Could you check a few things on this model? Use its own coordinates, in mm. A direction names the side the tool comes from. Coordinates: 2 decimals unless noted, no trailing zeros. Loops run counter-clockwise (first coordinate to the right, second up) from the corner with the lowest first, then second, coordinate; pieces in that order, holes last. Notation, with made-up numbers: (-14, 60.5) -> (44, 60.5) arc R22 ccw to (44, 89.5) -> close; hole circle Ø9 at (-26.75, -5). An arc over 180 degrees is marked (long way). One line per question, with ' | ' between items.
Autodesk Fusion 360 part; units mm, degrees
sketch "Sketch2" plane through (0, 0, 0) normal (0, 0, 1) x (1, 0, 0)
  line L0 (0, 0) -> (146.5, 0)
  line L1 (146.5, 0) -> (146.5, 57.5)
  line L2 (146.5, 57.5) -> (0, 57.5)
  line L3 (0, 57.5) -> (0, 0)
  line L4 (69.25, 0) -> (77.25, 0)
  line L5 (77.25, 0) -> (77.25, -8)
  line L6 (77.25, -8) -> (69.25, -8)
  line L7 (69.25, -8) -> (69.25, 0)
  line L8 (146.5, 24.75) -> (146.5, 32.75)
  line L9 (146.5, 32.75) -> (154.5, 32.75)
  line L10 (154.5, 32.75) -> (154.5, 24.75)
  line L11 (154.5, 24.75) -> (146.5, 24.75)
  line L12 (73.25, 57.5) -> (73.25, 0) construction
  line L13 (146.5, 28.75) -> (154.5, 28.75) construction
  line L14 (150.5, 32.75) -> (150.5, 24.75) construction
  circle A0 centre (150.5, 28.75) radius 1.75
  line L15 (-8, 24.75) -> (0, 24.75)
  line L16 (-8, 32.75) -> (-8, 24.75)
  line L17 (0, 32.75) -> (-8, 32.75)
  circle A1 centre (-4, 28.75) radius 1.75
  line L18 (69.25, -4) -> (77.25, -4) construction
  line L19 (73.25, 0) -> (73.25, -8) construction
  circle A2 centre (73.25, -4) radius 1.75
  point P0 (73.25, 0)
  point P1 (146.5, 28.75)
  point P2 (-8, 28.75)
  dimension "d8" = 146.5
  dimension "d9" = 57.5
  dimension "d12" = 8
  dimension "d13" = 8
  dimension "d14" = 8
  dimension "d15" = 8
  dimension "d16" = 8
  dimension "d17" = 3.5
  dimension "d18" = 3.5
extrude "Extrude1" add sketch "Sketch2" along normal blind 3
fillet "Fillet1" radius 1.5 12 edges at (77.25, 0, 1.5) (77.25, -8, 1.5) (69.25, -8, 1.5) (69.25, 0, 1.5) (0, 24.75, 1.5) (-8, 24.75, 1.5) (-8, 32.75, 1.5) (0, 32.75, 1.5) (154.5, 32.75, 1.5) (146.5, 32.75, 1.5) (146.5, 24.75, 1.5) (154.5, 24.75, 1.5)
sketch "Sketch3" plane through (0, 0, 3) normal (0, 0, 1) x (-1, 0, 0)
  arc A0 (-153, -24.75) -> (-154.5, -26.25) centre (-153, -26.25) ccw
  line L0 (-154.5, -26.25) -> (-154.5, -31.25)
  arc A1 (-154.5, -31.25) -> (-153, -32.75) centre (-153, -31.25) ccw
  line L1 (-153, -32.75) -> (-148, -32.75)
  arc A2 (-146.5, -34.25) -> (-148, -32.75) centre (-148, -34.25) ccw
  line L2 (-146.5, -34.25) -> (-146.5, -57.5)
  line L3 (-146.5, -57.5) -> (0, -57.5)
  line L4 (0, -57.5) -> (0, -34.25)
  arc A3 (1.5, -32.75) -> (0, -34.25) centre (1.5, -34.25) ccw
  line L5 (1.5, -32.75) -> (6.5, -32.75)
  arc A4 (6.5, -32.75) -> (8, -31.25) centre (6.5, -31.25) ccw
  line L6 (8, -31.25) -> (8, -26.25)
  arc A5 (8, -26.25) -> (6.5, -24.75) centre (6.5, -26.25) ccw
  line L7 (6.5, -24.75) -> (1.5, -24.75)
  arc A6 (0, -23.25) -> (1.5, -24.75) centre (1.5, -23.25) ccw
  line L8 (0, -23.25) -> (0, 0)
  line L9 (0, 0) -> (-67.75, 0)
  arc A7 (-69.25, 1.5) -> (-67.75, 0) centre (-67.75, 1.5) ccw
  line L10 (-69.25, 1.5) -> (-69.25, 6.5)
  arc A8 (-69.25, 6.5) -> (-70.75, 8) centre (-70.75, 6.5) ccw
  line L11 (-70.75, 8) -> (-75.75, 8)
  arc A9 (-75.75, 8) -> (-77.25, 6.5) centre (-75.75, 6.5) ccw
  line L12 (-77.25, 6.5) -> (-77.25, 1.5)
  arc A10 (-78.75, 0) -> (-77.25, 1.5) centre (-78.75, 1.5) ccw
  line L13 (-78.75, 0) -> (-146.5, 0)
  line L14 (-146.5, 0) -> (-146.5, -23.25)
  arc A11 (-148, -24.75) -> (-146.5, -23.25) centre (-148, -23.25) ccw
  line L15 (-148, -24.75) -> (-153, -24.75)
  circle A12 centre (-150.5, -28.75) radius 1.75
  circle A13 centre (4, -28.75) radius 1.75
  circle A14 centre (-73.25, 4) radius 1.75
  line L16 (0, -2.5) -> (-146.5, -2.5) construction
  line L17 (-54.25, -2.5) -> (-92.25, -2.5)
  line L18 (-92.25, -2.5) -> (-92.25, 0)
  line L19 (-54.25, -2.5) -> (-54.25, 0)
  line L20 (-54.25, 0) -> (-92.25, 0)
  line L21 (-144, -57) -> (-144, 0) construction
  line L22 (-144, -13.5) -> (-144, -43.5)
  line L23 (-144, -43.5) -> (-146.5, -43.5)
  line L24 (-144, -13.5) -> (-146.5, -13.5)
  line L25 (-146.5, -13.5) -> (-146.5, -43.5)
  line L26 (-73.25, -57.5) -> (-73.25, 0) construction
  line L27 (-2.5, -13.5) -> (0, -13.5)
  line L28 (0, -13.5) -> (0, -43.5)
  line L29 (-2.5, -43.5) -> (0, -43.5)
  line L30 (-2.5, -13.5) -> (-2.5, -43.5)
  line L31 (0, -55) -> (-146.5, -55) construction
  line L32 (-50.75, -55) -> (-95.75, -55)
  line L33 (-95.75, -55) -> (-95.75, -57.5)
  line L34 (-50.75, -55) -> (-50.75, -57.5)
  line L35 (-50.75, -57.5) -> (-95.75, -57.5)
  line L36 (-70.75, -55) -> (-75.75, -55)
  line L37 (-75.75, -55) -> (-75.75, -57.5)
  line L38 (-75.75, -57.5) -> (-70.75, -57.5)
  line L39 (-70.75, -57.5) -> (-70.75, -55)
  point P0 (-73.25, -2.5)
  point P1 (-144, -28.5)
  point P2 (-73.25, -55)
  point P3 (-73.25, -55)
  dimension "d23" = 2.5
  dimension "d24" = 38
  dimension "d25" = 2.5
  dimension "d26" = 30
  dimension "d27" = 2.5
  dimension "d28" = 45
  dimension "d29" = 5
extrude "Extrude2" add sketch "Sketch3" along normal blind 10 contours L2 L14 L22 L23 L24 L25 | L9 L13 L17 L18 L19 L20 | L3 L32 L33 L35 L37 | L3 L32 L34 L35 L39 | L4 L8 L27 L28 L29 L30
equation "controller_length = 143 mm"
equation "controller_width = 54 mm"
equation "mount_hole_diameter = 3.5 mm"
equation "base_thickness = 3 mm"
equation "wall_thickness = 2.5 mm"
equation "give = 1 mm"
equation "d8 = total_length"
equation "d9 = total_width"
equation "total_length = controller_length + wall_thickness + give"
equation "total_width = controller_width + give + wall_thickness"
equation "d19 = base_thickness"
equation "d23 = wall_thickness"
equation "d25 = wall_thickness"
equation "d27 = wall_thickness"
1) If we section it at B-B on x = 150.5: Please give me the cut outline in (y, z), and give its area (3 significant figures).
Data:
outline: (24.75, 0) -> (27, 0) -> (27, 3) -> (24.75, 3) -> close; (30.5, 0) -> (32.75, 0) -> (32.75, 3) -> (30.5, 3) -> close | area: 13.5 mm²
2) I need wall thicknesses on line 1 along Y through (x, z) = (150.5, 1.65); line 2 along X through (y, z) = (32.5, 11.75); line 3 along Y through (x, z) = (73.25, 0.85). Which ranges of each line are inside material? Lowest first, please. Write a range as from..to.
Data:
line 1: 24.75..27, 30.5..32.75 | line 2: 0..2.5, 144..146.5 | line 3: -8..-5.75, -2.25..57.5
3) On a 3-axis mill with a long thin cutter (end or side, diameter ignored), from which of +Z, -Z, +X, -X, +Y, -Y can I reach the whole of each face in a straight line? I mean faces 1 (the face through (148.7, 27.6, 3)), 2 (the face through (150, 32.75, 1)), 3 (the face through (69.25, -4, 1)), 4 (the face through (77.25, -4, 1)), 5 (the face through (144, 28, 8)). Say none if no direction works.
Data:
face 1: +Z, +X, +Y, -Y | face 2: +Z, -Z, +X, +Y | face 3: +Z, -Z, -X, -Y | face 4: +Z, -Z, +X, -Y | face 5: +Z, +Y, -Y
4) We'd pull the mould along Y, two halves only. Please class faces 6 (the face through (-5.75, 28.67, 1.48)), 7 (the face through (61, 55, 8)), 8 (the face through (72, 0, 5)), 9 (the face through (-6, 29, 3)): pulls with the +Y half, pulls with the -Y half, needs draft (parallel to the pull), parting line crosses it, or undercut.
Data:
face 6: undercut | face 7: undercut | face 8: pulls with the -Y half | face 9: needs draft
5) If we section it at D-D on y = 41.5: Please give me the cut outline in (x, z).
Data:
outline: (0, 0) -> (146.5, 0) -> (146.5, 13) -> (144, 13) -> (144, 3) -> (2.5, 3) -> (2.5, 13) -> (0, 13) -> close
6) If we section it at A-A on y = -4: Please give me the cut outline in (x, z), and give its area (3 significant figures).
Data:
outline: (69.25, 0) -> (71.5, 0) -> (71.5, 3) -> (69.25, 3) -> close; (75, 0) -> (77.25, 0) -> (77.25, 3) -> (75, 3) -> close | area: 13.5 mm²
7) I'm going to push flat-ended pins straight in: pin 1 Ø9 at (x, y) = (-5.5, 31.5) entering from +Z; pin 2 Ø3 at (y, z) = (56.5, 10) entering from +X; pin 3 Ø3 at (x, y) = (150.5, 28.75) entering from -Z; pin 4 Ø3.5 at (y, z) = (-5, 1) entering from -X. Where does each tip first touch, or does it pass through?
Data:
pin 1: z = 3 | pin 2: x = 95.75 | pin 3: through | pin 4: x = 69.25
8) If we section it at C-C on z = 7: Please give me the cut outline in (x, y), and give its area (3 significant figures).
Data:
outline: (0, 13.5) -> (2.5, 13.5) -> (2.5, 43.5) -> (0, 43.5) -> close; (50.75, 55) -> (70.75, 55) -> (70.75, 57.5) -> (50.75, 57.5) -> close; (54.25, 0) -> (92.25, 0) -> (92.25, 2.5) -> (54.25, 2.5) -> close; (75.75, 55) -> (95.75, 55) -> (95.75, 57.5) -> (75.75, 57.5) -> close; (144, 13.5) -> (146.5, 13.5) -> (146.5, 43.5) -> (144, 43.5) -> close | area: 345 mm²
